```python
from build123d import *

# Parameters (mm, degrees)
SKETCH19_W          = 20
SKETCH19_H          = 10
BOSS_EXTRUDE4_DEPTH = 3
SKETCH22_R          = 2.5
BOSS_EXTRUDE5_DEPTH = 3


with BuildPart() as part:
    # Sketch19 → Boss-Extrude4 (new body)
    with BuildSketch(Plane.XY):
        Rectangle(SKETCH19_W, SKETCH19_H)
    boss_extrude4 = extrude(amount=-BOSS_EXTRUDE4_DEPTH)

    # Sketch22 → Boss-Extrude5 (add)
    with BuildSketch(Plane.XY):
        with BuildLine():
            Line((10, 5), (20, 5))
            ThreePointArc((20, 5), (25, 0), (20, -5))
            Line((20, -5), (10, -5))
            Line((10, -5), (10, 5))
        make_face()
        with Locations((20, 0)):
            Circle(SKETCH22_R, mode=Mode.SUBTRACT)
    boss_extrude5 = extrude(amount=-BOSS_EXTRUDE5_DEPTH)

    # Mirror2: Boss-Extrude4, Boss-Extrude5 across plane
    add(boss_extrude4.mirror(Plane.ZY))
    add(boss_extrude5.mirror(Plane.ZY))


solid = part.part
```
CAD build for the part. Positions are in the model's coordinates, mm. Coordinates: 2 decimals unless noted, no trailing zeros. Write each loop counter-clockwise with the first axis right and the second up, starting at its lowest first coordinate (ties: lowest second). Pieces come first, ordered by that corner, then holes. Notation, with made-up numbers: (51.5, 0) -> (68.5, 0) arc R17 cw to (68.5, 12) -> close; hole circle Ø1 at (50.25, 67). An arc over 180 degrees is marked (long way). Return JSON: item names as keys, results as strings. Group by question number.
Q1. Cut at D-D, the plane y = -3. Give the cut face in (x, z), then the cut area to 3 significant figures.
Q2. Cut at A-A, the plane y = 0. Give the cut face in (x, z).
Q3. Pull direction Y, two halves, no side cores. Call faces 1 (the face through (0, 0, 0)), 2 (the face through (0, -5, -1)), 3 (the face through (17.5, 0.1, -1.5)): released by +Y, released by -Y, zero draft, split by the parting line, or undercut.
Q4. Drill centre lines: line 1 (X direction, y = -1.5, z = -2.1); line 2 (X direction, y = 1, z = -1.15); line 3 (Y direction, x = 20, z = -1.65). Where is each one in solid material? Low to high.
Q5. Cut at C-C, the plane z = -0.5. Give the cut face in (x, y).
Q6. Cut at B-B, the plane x = -19. Give the cut face in (y, z), then the cut area to 3 significant figures.
Returned:
{
 "1": {"outline": "(-24, -3) -> (24, -3) -> (24, 0) -> (-24, 0) -> close", "area": "144 mm2"},
 "2": {"outline": "(-25, -3) -> (-22.5, -3) -> (-22.5, 0) -> (-25, 0) -> close; (-17.5, -3) -> (17.5, -3) -> (17.5, 0) -> (-17.5, 0) -> close; (22.5, -3) -> (25, -3) -> (25, 0) -> (22.5, 0) -> close"},
 "3": {"face 1": "zero draft", "face 2": "released by -Y", "face 3": "undercut"},
 "4": {"line 1": "x = -24.77 to -22, -18 to 18, 22 to 24.77", "line 2": "x = -24.9 to -22.29, -17.71 to 17.71, 22.29 to 24.9", "line 3": "y = -5 to -2.5, 2.5 to 5"},
 "5": {"outline": "(-20, -5) -> (20, -5) arc R5 ccw to (20, 5) -> (-20, 5) arc R5 ccw to start; hole circle Ø5 at (-20, 0); hole circle Ø5 at (20, 0)"},
 "6": {"outline": "(-5, -3) -> (-2.29, -3) -> (-2.29, 0) -> (-5, 0) -> close; (2.29, -3) -> (5, -3) -> (5, 0) -> (2.29, 0) -> close", "area": "16.3 mm2"}
}
